```python
from build123d import *

# Parameters (mm, degrees)
F1_DEPTH = 7
F2_R     = 6.5
F2_W     = 7.5
F2_H     = 7.5
F3_DEPTH = 15
F2_R_2   = 2
F4_DEPTH = 25
F5_START = -5
F5_DEPTH = 10.001
F6_R     = 2
F7_DEPTH = 2.8


with BuildPart() as f1:
    # F0 (on Top) → F1 (new body)
    with BuildSketch(Plane.XY):
        with BuildLine():
            Line((45.3333333333, 4.9888765157), (0.5333333333, 7.9822024251))
            ThreePointArc((0.5333333333, 7.9822024251), (-8, 0), (0.5333333333, -7.9822024251))
            Line((0.5333333333, -7.9822024251), (45.3333333333, -4.9888765157))
            ThreePointArc((45.3333333333, -4.9888765157), (50, 0), (45.3333333333, 4.9888765157))
        make_face()
    extrude(amount=F1_DEPTH)

    # F2 (on face) → F3 (join)
    with BuildSketch(Plane.XY.offset(7)):
        Circle(F2_R)
        Rectangle(F2_W, F2_H, mode=Mode.SUBTRACT)
    extrude(amount=-F3_DEPTH)

    # F2 (on face) → F4 (cut)
    with BuildSketch(Plane.XY.offset(7)):
        with Locations((45, 0)):
            Circle(F2_R_2)
    extrude(amount=-F4_DEPTH, mode=Mode.SUBTRACT)

    # F2 (on face) → F5 (cut)
    with BuildSketch(Plane.XY.offset(7).offset(F5_START)):
        Rectangle(F2_W, F2_H)
    extrude(amount=-F5_DEPTH, mode=Mode.SUBTRACT)

    # F6
    f6_edges = [f1.edges().sort_by_distance(p)[0] for p in [
        (22.933333, -6.485539, 7),
        (22.933333, 6.485539, 0),
    ]]
    fillet(f6_edges, radius=F6_R)

    # F2 (on face) → F7 (join)
    with BuildSketch(Plane.XY.offset(7)):
        with BuildLine():
            ThreePointArc((45.3333333333, -4.9888765157), (48.6514837167, -3.4156502553), (50, 0))
            ThreePointArc((50, 0), (48.6514837167, 3.4156502553), (45.3333333333, 4.9888765157))
            ThreePointArc((45.3333333333, 4.9888765157), (40, 0), (45.3333333333, -4.9888765157))
        make_face()
        with Locations((45, 0)):
            Circle(F2_R_2, mode=Mode.SUBTRACT)
    extrude(amount=-F7_DEPTH)


solid = f1.part
```
Part model, mm, in its own coordinate system. A direction names the side the tool comes from. Coordinates: 2 decimals unless noted, no trailing zeros. Order: outer loops, then holes, each group sorted by start corner. A loop starts at its lowest first (then second) coordinate and runs counter-clockwise, first axis right, second up. Notation, with made-up numbers: (-39, -7.5) -> (4, -7.5) arc R18 ccw to (4, 3.5) -> close; hole circle Ø6 at (32.5, -19.75). An arc over 180 degrees is marked (long way). Put each result on its own line as item: value. Start each with the question number.
(1) Band-saw the part on B-B (z = 4). Give the cut face in (x, y), then the cut area to 3 significant figures.
(2) Band-saw the part on C-C (z = 1.25). Count the separate pieces of the cut face and the enclosed holes in it, then the cut area to 3 significant figures.
(3) Band-saw the part on A-A (z = -2). Give the cut face in (x, y), then the cut area to 3 significant figures.
(4) Pin check, flat tips, straight feed: pin 1 Ø6 at (y, z) = (4, -1.5) entering from -X; pin 2 Ø2 at (y, z) = (1, -2) entering from -X; pin 3 Ø6 at (y, z) = (-1.5, -2) entering from +X. Stop position of each tip, or through.
(5) Probe line 1 along Y through (x, z) = (45, 5.75); line 2 along X through (y, z) = (0.5, -6); line 3 along Z through (x, y) = (27, -0.75). List the from-to ranges inside material, lowest first. Write a range as [from, to].
(6) Mould opens along Y. For faces 1 (the face through (0, -4, -8)), 2 (the face through (22.62, -6.506, 3.447)), 3 (the face through (23.247, 6.465, 3.447)), 4 (the face through (0, 3.75, -3)) say: pulls with the +Y half, pulls with the -Y half, needs draft (parallel to the pull), parting line crosses it, or undercut.
(7) Which spindle directions (+Z, -Z, +X, -X, +Y, -Y) get a long thin tool onto all of the face, cutting with end or side? Do faces 5 (the face through (0, 0, 2)), 6 (the face through (23.207, -5.865, 6.43)), 7 (the face through (22.58, 5.906, 6.43)). Say none if no direction does.
Determined:
1. outline: (0.53, -7.98) -> (45.33, -4.99) arc R5 ccw to (45.33, 4.99) -> (0.53, 7.98) arc R8 ccw (long way) to start; hole circle Ø4 at (45, 0)
1. area: 714 mm²
2. separate pieces: 1
2. enclosed holes: 2
2. area: 639 mm²
3. outline: circle Ø13 at (0, 0); hole (-3.75, -3.75) -> (3.75, -3.75) -> (3.75, 3.75) -> (-3.75, 3.75) -> close
3. area: 76.5 mm²
4. pin 1: stops at x = -7.41
4. pin 2: stops at x = -6.5
4. pin 3: stops at x = 49.61
5. line 1: y = [-5, -2], [2, 5]
5. line 2: x = [-6.48, -3.75], [3.75, 6.48]
5. line 3: z = [0, 7]
6. face 1: needs draft
6. face 2: pulls with the -Y half
6. face 3: pulls with the +Y half
6. face 4: undercut
7. face 5: -Z
7. face 6: +Z, -Y
7. face 7: +Z, +Y
